Part model, mm, in its own coordinate system. A direction names the side the tool comes from. Coordinates: 2 decimals unless noted, no trailing zeros. Write each loop counter-clockwise with the first axis right and the second up, starting at its lowest first coordinate (ties: lowest second). Pieces come first, ordered by that corner, then holes. Notation, with made-up numbers: (-33.75, 31) -> (-18.75, 31) arc R16 ccw to (-18.75, 38) -> close; hole circle Ø5 at (-6.5, 17). An arc over 180 degrees is marked (long way). One line per question, with ' | ' between items. Start each with the question number.
Item 1: Probe probe 1 along X at (y, z) = (0.75, 10.5); probe 2 along Y at (x, z) = (-11, 5); probe 3 along Z at (x, y) = (-3, -1.25) (3 decimals). List the from-to ranges inside material, lowest first. Write a range as [from, to].
Item 2: Saw through at C-C (z = 4). List the corners of the cut face in (x, y), and give its area (3 significant figures).
Item 3: Two-plate mould, pull along X, no slides. Class faces 4 (the flat face through (-25.7, -2, -11)), 5 (the flat face through (0, 4.63, 12)), 6 (the cylindrical face through (-27.513, 0.826, -12.07)): pulls with the +X half, pulls with the -X half, needs draft (parallel to the pull), parting line crosses it, or undercut.
Item 4: Saw through at D-D (y = -2.5). List the corners of the cut face in (x, z) (3 decimals), and give its area (3 significant figures).
Item 5: Saw through at A-A (y = 3). List the corners of the cut face in (x, z) (3 decimals).
Item 6: Pin check, flat tips, straight feed: pin 1 (3.5 mm diameter, centred on x = 29, z = -11.875, fed in from -Y); pin 2 (3 mm diameter, centred on y = 6, z = 9, fed in from +X); pin 3 (1.8 mm diameter, centred on x = -29, z = 11.875, fed in from -Y); pin 4 (2.5 mm diameter, centred on y = 4, z = 12.5, fed in from -X). Stop position of each tip, or through.
Item 7: 3-axis set-ups, long thin cutter, end or side, ignore diameter. For faces 1 (the flat face through (8.5, 3, 12)), 2 (the flat face through (0, 3, 9.284)), 3 (the flat face through (-8.5, 3, 12)): which of +Z, -Z, +X, -X, +Y, -Y reach the whole face in a straight line?
Item 8: Saw through at B-B (x = -1.5). List the corners of the cut face in (y, z) (3 decimals).
from build123d import *

# Parameters (mm, degrees)
EXTRUDE_1_DEPTH     = 1.63
SKETCH_2_R          = 1.5
CUT_EXTRUDE_1_DEPTH = 2.63
SKETCH_8_W          = 51
SKETCH_8_H          = 5
EXTRUDE_6_DEPTH     = 3.68
SKETCH_9_W          = 17
SKETCH_9_H          = 6.090540171
EXTRUDE_7_DEPTH     = 3
SKETCH_10_W         = 20
SKETCH_10_H         = 6
EXTRUDE_8_DEPTH     = 6


with BuildPart() as part:
    # 草图1 → 凸台-拉伸1 (new body)
    with BuildSketch(Plane(origin=(0, 0, 0), x_dir=(1, 0, 0), z_dir=(0, 1, 0))):
        with BuildLine():
            Line((-29.5, 15.375), (29.5, 15.375))
            ThreePointArc((29.5, 15.375), (31.621320344, 14.496320344), (32.5, 12.375))
            Line((32.5, 12.375), (32.5, -12.375))
            ThreePointArc((32.5, -12.375), (31.621320344, -14.496320344), (29.5, -15.375))
            Line((29.5, -15.375), (-29.5, -15.375))
            ThreePointArc((-29.5, -15.375), (-31.621320344, -14.496320344), (-32.5, -12.375))
            Line((-32.5, -12.375), (-32.5, 12.375))
            ThreePointArc((-32.5, 12.375), (-31.621320344, 14.496320344), (-29.5, 15.375))
        make_face()
    extrude(amount=EXTRUDE_1_DEPTH)

    # 草图2 → 切除-拉伸1 (cut, through all)
    with BuildSketch(Plane(origin=(0, 1.63, 0), x_dir=(1, 0, 0), z_dir=(0, 1, 0))):
        with Locations(Location((-29, 11.875, 0), (0, 0, 270))):  # turned: the seam where the file's is
            Circle(SKETCH_2_R)
        with Locations(Location((-29, -11.875, 0), (0, 0, 270))):  # turned: the seam where the file's is
            Circle(SKETCH_2_R)
        with Locations(Location((29, -11.875, 0), (0, 0, 270))):  # turned: the seam where the file's is
            Circle(SKETCH_2_R)
        with Locations(Location((29, 11.875, 0), (0, 0, 270))):  # turned: the seam where the file's is
            Circle(SKETCH_2_R)
    extrude(amount=-CUT_EXTRUDE_1_DEPTH, mode=Mode.SUBTRACT)

    # 草图8 → 凸台-拉伸6 (add)
    with BuildSketch(Plane.XZ):
        with Locations((-0.2, -11.235)):
            Rectangle(SKETCH_8_W, SKETCH_8_H)
    extrude(amount=EXTRUDE_6_DEPTH)

    # 草图9 → 凸台-拉伸7 (add)
    with BuildSketch(Plane(origin=(0, 1.63, 0), x_dir=(1, 0, 0), z_dir=(0, 1, 0))):
        with Locations((0, -12.329729915)):
            Rectangle(SKETCH_9_W, SKETCH_9_H)
    extrude(amount=EXTRUDE_7_DEPTH)

    # 草图10 → 凸台-拉伸8 (add)
    with BuildSketch(Plane(origin=(0, 1.63, 0), x_dir=(1, 0, 0), z_dir=(0, 1, 0))):
        with Locations((0, 12.375)):
            Rectangle(SKETCH_10_W, SKETCH_10_H)
    extrude(amount=EXTRUDE_8_DEPTH)


solid = part.part
From the geometry:
1) probe 1: [-32.5, -29.6], [-28.4, 28.4], [29.6, 32.5] | probe 2: [0, 1.63] | probe 3: [-13.735, -8.735]
2) outline: (-32.5, 0) -> (32.5, 0) -> (32.5, 1.63) -> (-32.5, 1.63) -> close | area: 106 mm2
3) face 4: pulls with the -X half | face 5: needs draft | face 6: undercut
4) outline: (-25.7, -13.735) -> (25.3, -13.735) -> (25.3, -8.735) -> (-25.7, -8.735) -> close | area: 255 mm2
5) outline: (-10, -15.375) -> (10, -15.375) -> (10, -9.375) -> (-10, -9.375) -> close; (-8.5, 9.284) -> (8.5, 9.284) -> (8.5, 15.375) -> (-8.5, 15.375) -> close
6) pin 1: y = 0 | pin 2: x = 8.5 | pin 3: through | pin 4: x = -8.5
7) face 1: +Z, +X, +Y | face 2: +X, -X, +Y | face 3: +Z, -X, +Y
8) outline: (-3.68, -13.735) -> (0, -13.735) -> (0, -15.375) -> (7.63, -15.375) -> (7.63, -9.375) -> (1.63, -9.375) -> (1.63, 9.284) -> (4.63, 9.284) -> (4.63, 15.375) -> (0, 15.375) -> (0, -8.735) -> (-3.68, -8.735) -> close
